Geometry: final body of the model. Coordinates: model frame, mm. Give positions to 0.01 mm unless a question says otherwise; leave off trailing zeros. Order: outer loops, then holes, each group sorted by start corner. A loop starts at its lowest first (then second) coordinate and runs counter-clockwise, first axis right, second up. Notation, with made-up numbers: (59.25, 53.5) - (103.25, 53.5) arc R23 ccw to (103.25, 63.5) - close; hole circle Ø10 at (-8.75, -8.5). An arc over 180 degrees is marked (long way). One line per item, written item: value.
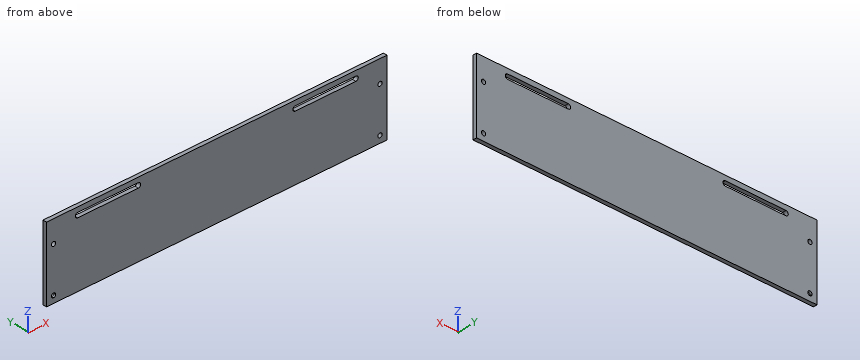
```python
from build123d import *

# Parameters (mm, degrees)
F0_R     = 1.75
F1_DEPTH = 1.5875


with BuildPart() as f1:
    # F0 (on Front) → F1 (new body, symmetric)
    with BuildSketch(Plane.XZ):
        with BuildLine():
            Line((140.3, -30.48), (140.3, 30.48))
            Line((140.3, 30.48), (-140.3, 30.48))
            Line((-140.3, 30.48), (-140.3, -24.68))
            Line((-140.3, -24.68), (-136.25, -24.68))
            ThreePointArc((-136.25, -24.68), (-134.5, -22.93), (-132.75, -24.68))
            ThreePointArc((-132.75, -24.68), (-133.2625631329, -25.9174368671), (-134.5, -26.43))
            Line((-134.5, -26.43), (-134.5, -30.48))
            Line((-134.5, -30.48), (140.3, -30.48))
        make_face()
        with Locations((134.5, -24.68)):
            Circle(F0_R, mode=Mode.SUBTRACT)
        with Locations((-134.5, 12.32)):
            Circle(F0_R, mode=Mode.SUBTRACT)
        with BuildLine():
            Line((-114.69375, 26.44616), (-89.69375, 26.44616))
            Line((-89.69375, 26.44616), (-64.69375, 26.44616))
            ThreePointArc((-64.69375, 26.44616), (-62.76875, 24.52116), (-64.69375, 22.59616))
            Line((-64.69375, 22.59616), (-89.69375, 22.59616))
            Line((-89.69375, 22.59616), (-114.69375, 22.59616))
            ThreePointArc((-114.69375, 22.59616), (-116.61875, 24.52116), (-114.69375, 26.44616))
        make_face(mode=Mode.SUBTRACT)
        with Locations((134.5, 12.32)):
            Circle(F0_R, mode=Mode.SUBTRACT)
        with BuildLine():
            ThreePointArc((64.69375, 22.59616), (62.76875, 24.52116), (64.69375, 26.44616))
            Line((64.69375, 26.44616), (114.69375, 26.44616))
            ThreePointArc((114.69375, 26.44616), (116.61875, 24.52116), (114.69375, 22.59616))
            Line((114.69375, 22.59616), (64.69375, 22.59616))
        make_face(mode=Mode.SUBTRACT)
        with BuildLine():
            Line((-136.25, -24.68), (-140.3, -24.68))
            Line((-140.3, -24.68), (-140.3, -30.48))
            Line((-140.3, -30.48), (-134.5, -30.48))
            Line((-134.5, -30.48), (-134.5, -26.43))
            ThreePointArc((-134.5, -26.43), (-135.7374368671, -25.9174368671), (-136.25, -24.68))
        make_face()
    extrude(amount=F1_DEPTH, both=True)


solid = f1.part
```
1) First-contact query: pin 1 (3 mm diameter, centred on x = 134.5, z = -24.68, fed in from +Y). Flat tip, straight axial feed; report the tip coordinate or a pass-through.
Answers below:
pin 1: through
2) Section B-B, the plane x = -96.5. Return loops of the section in (y, z).
Answers below:
outline: (-1.59, -30.48) - (1.59, -30.48) - (1.59, 22.6) - (-1.59, 22.6) - close; (-1.59, 26.45) - (1.59, 26.45) - (1.59, 30.48) - (-1.59, 30.48) - close
3) Section A-A, the plane y = -0.8. Return loops of the section in (x, z) (3 decimals), then the cut area to 3 significant figures.
Answers below:
outline: (-140.3, -30.48) - (140.3, -30.48) - (140.3, 30.48) - (-140.3, 30.48) - close; hole circle Ø3.5 at (-134.5, -24.68); hole circle Ø3.5 at (-134.5, 12.32); hole (-114.694, 22.596) - (-64.694, 22.596) arc R1.925 ccw to (-64.694, 26.446) - (-114.694, 26.446) arc R1.925 ccw to start; hole (64.694, 22.596) - (114.694, 22.596) arc R1.925 ccw to (114.694, 26.446) - (64.694, 26.446) arc R1.925 ccw to start; hole circle Ø3.5 at (134.5, -24.68); hole circle Ø3.5 at (134.5, 12.32)
area: 16,700 mm^2
4) Material intervals for line 1 along Z through (x, y) = (134.5, 0.15); line 2 along Z through (x, y) = (72.5, 0.8); line 3 along X through (y, z) = (0.5, -25.5), sorted ascending.
Answers below:
line 1: -30.48 to -26.43, -22.93 to 10.57, 14.07 to 30.48
line 2: -30.48 to 22.6, 26.45 to 30.48
line 3: -140.3 to -136.05, -132.95 to 132.95, 136.05 to 140.3
